Check sheet for the modelled part. Datum: model origin and axes. Units: mm. A direction names the side the tool comes from. Give positions to 0.01 mm unless a question says otherwise; leave off trailing zeros. Loops run counter-clockwise (first coordinate to the right, second up) from the corner with the lowest first, then second, coordinate; pieces in that order, holes last. Notation, with made-up numbers: (2, 23.25) - (51, 23.25) arc R11 cw to (51, 41.25) - close; hole circle Ø8 at (26, 38.25). An arc over 180 degrees is marked (long way). Use one line per item in the form item = value.
from build123d import *

# Parameters (mm, degrees)
F0_W     = 47
F0_H     = 29
F1_DEPTH = 3
F0_R     = 1.65
F2_DEPTH = 3
F3_W     = 41
F3_H     = 23
F4_DEPTH = 3.001


with BuildPart() as f1:
    # F0 (on Top) → F1 (new body)
    with BuildSketch(Plane.XY):
        with Locations((0, 14.5)):
            Rectangle(F0_W, F0_H)
    extrude(amount=F1_DEPTH)

    # F0 (on Top) → F2 (join)
    with BuildSketch(Plane.XY):
        with BuildLine():
            ThreePointArc((-21.533361, 33.65), (-23.10973, 33.904996), (-24.525312, 34.643976))
            ThreePointArc((-24.525312, 34.643976), (-28.834444, 34.33246), (-29.142296, 30.023065))
            ThreePointArc((-29.142296, 30.023065), (-28.401441, 28.606095), (-28.145774, 27.027708))
            Line((-28.145774, 27.027708), (-28.145774, 1.972292))
            ThreePointArc((-28.145774, 1.972292), (-28.401441, 0.393905), (-29.142296, -1.023065))
            ThreePointArc((-29.142296, -1.023065), (-29.617954, -4.080909), (-27.351685, -6.188202))
            ThreePointArc((-27.351685, -6.188202), (-25.876037, -6.240474), (-24.525312, -5.643976))
            ThreePointArc((-24.525312, -5.643976), (-23.10973, -4.904996), (-21.533361, -4.65))
            Line((-21.533361, -4.65), (21.533361, -4.65))
            ThreePointArc((21.533361, -4.65), (23.10973, -4.904996), (24.525312, -5.643976))
            ThreePointArc((24.525312, -5.643976), (25.876037, -6.240474), (27.351685, -6.188202))
            ThreePointArc((27.351685, -6.188202), (29.617954, -4.080909), (29.142296, -1.023065))
            ThreePointArc((29.142296, -1.023065), (28.401441, 0.393905), (28.145774, 1.972292))
            Line((28.145774, 1.972292), (28.145774, 27.027708))
            ThreePointArc((28.145774, 27.027708), (28.401441, 28.606095), (29.142296, 30.023065))
            ThreePointArc((29.142296, 30.023065), (28.834444, 34.33246), (24.525312, 34.643976))
            ThreePointArc((24.525312, 34.643976), (23.10973, 33.904996), (21.533361, 33.65))
            Line((21.533361, 33.65), (-21.533361, 33.65))
        make_face()
        with Locations((-26.5, -3)):
            Circle(F0_R, mode=Mode.SUBTRACT)
        with Locations((26.5, -3)):
            Circle(F0_R, mode=Mode.SUBTRACT)
        with BuildLine():
            ThreePointArc((-28.145774, 32.118016), (-26.440954, 33.648943), (-24.85, 32))
            ThreePointArc((-24.85, 32), (-26.440954, 30.351057), (-28.145774, 31.881984))
            ThreePointArc((-28.145774, 31.881984), (-28.15, 32), (-28.145774, 32.118016))
        make_face(mode=Mode.SUBTRACT)
        with Locations((0, 14.5)):
            Rectangle(F0_W, F0_H, mode=Mode.SUBTRACT)
        with BuildLine():
            ThreePointArc((28.145774, 32.118016), (28.148943, 32.059046), (28.15, 32))
            ThreePointArc((28.15, 32), (28.148943, 31.940954), (28.145774, 31.881984))
            ThreePointArc((28.145774, 31.881984), (24.85, 32), (28.145774, 32.118016))
        make_face(mode=Mode.SUBTRACT)
    extrude(amount=F2_DEPTH)

    # F3 (on face) → F4 (cut, through all)
    with BuildSketch(Plane.XY.offset(3)):
        with Locations((0, 14.5)):
            Rectangle(F3_W, F3_H)
    extrude(amount=-F4_DEPTH, mode=Mode.SUBTRACT)


solid = f1.part
Item 1: Section check B-B on z = 2.05. Give the number of separate pieces and of enclosed holes in the cut face, then the cut area to 3 significant figures.
Answer block:
separate_pieces = 1
enclosed_holes = 5
area = 1,230 mm2
Item 2: Section check C-C on x = 26.5. Record the boundary of the cut face in (y, z).
Answer block:
outline = (-6.3, 0) - (-4.65, 0) - (-4.65, 3) - (-6.3, 3) - close; (-1.35, 0) - (30.35, 0) - (30.35, 3) - (-1.35, 3) - close; (33.65, 0) - (35.3, 0) - (35.3, 3) - (33.65, 3) - close
Item 3: Access from +Z, -Z, +X, -X, +Y, -Y to the whole of each face (thin tool, end or side, straight path). Record for faces 5 (the face through (28.4, 28.6, 1.5)), 6 (the face through (0, 3, 2)), 7 (the face through (23.1, 33.9, 1.5)), 8 (the face through (-28.4, 28.6, 1.5)).
Answer block:
face_5 = +Z, -Z, +X
face_6 = +Z, -Z
face_7 = +Z, -Z, +Y
face_8 = +Z, -Z, -X
Item 4: Mould release check, pull along Y, two halves, no side actions. Record for faces 1 (the face through (0, -4.65, 1)), 2 (the face through (-20.5, 14, 2)), 3 (the face through (-28.787, 34.379, 1.479)), 4 (the face through (0, 29, 3)): released by +Y, released by -Y, zero draft, split by the parting line, or undercut.
Answer block:
face_1 = released by -Y
face_2 = undercut
face_3 = undercut
face_4 = zero draft
Item 5: Gauge pin test, flat ends, axial feed: P1, Ø1.5, axis at x = -6.5, z = 1.5, coming from the +Y side; P2, Ø4.5, axis at x = -26.5, y = -3, coming from the +Z side; P3, Ø1, axis at x = 9, z = 0.5, coming from the -Y side; P4, Ø0.9, axis at y = 18, z = 1, coming from the +X side. Record the tip position at first contact, or that the pin passes through.
Answer block:
P1 = 33.65
P2 = 3
P3 = -4.65
P4 = 28.15
Item 6: Section check A-A on y = 23.5. Record the boundary of the cut face in (x, z), then the cut area to 3 significant figures.
Answer block:
outline = (-28.15, 0) - (-20.5, 0) - (-20.5, 3) - (-28.15, 3) - close; (20.5, 0) - (28.15, 0) - (28.15, 3) - (20.5, 3) - close
area = 45.9 mm2
Item 7: Section check D-D on x = -3. Record the boundary of the cut face in (y, z), then the cut area to 3 significant figures.
Answer block:
outline = (-4.65, 0) - (3, 0) - (3, 3) - (-4.65, 3) - close; (26, 0) - (33.65, 0) - (33.65, 3) - (26, 3) - close
area = 45.9 mm2
Item 8: Thickness scan on L1, parallel to Y at x = 26.5, z = 2.2; L2, parallel to Y at x = -16, z = 1; L3, parallel to X at y = 12.5, z = 2.4. Record the ranges inside material, lowest first.
Answer block:
L1 = -6.3 to -4.65, -1.35 to 30.35, 33.65 to 35.3
L2 = -4.65 to 3, 26 to 33.65
L3 = -28.15 to -20.5, 20.5 to 28.15
